Could you check a few things on this model? Use its own coordinates, in mm. Give positions to 0.01 mm unless a question says otherwise; leave off trailing zeros. Write each loop counter-clockwise with the first axis right and the second up, starting at its lowest first coordinate (ties: lowest second). Pieces come first, ordered by that corner, then holes. Notation, with made-up numbers: M -38.75,-17 L 16.25,-17 A13 cw 16.25,2 Z; hole C 51.25,77.25 d3. An arc over 180 degrees is marked long. Answer as a JSON object with one key per item and string values. Group by question number.
```python
from build123d import *

# Parameters (mm, degrees)
SKETCH1_W           = 60
SKETCH1_H           = 45
SKETCH1_R           = 2
BOSS_EXTRUDE1_DEPTH = 2
SKETCH2_R           = 12
CUT_EXTRUDE1_DEPTH  = 38.553295461


with BuildPart() as part:
    # Sketch1 → Boss-Extrude1 (new body)
    with BuildSketch(Plane(origin=(0, 0, 0), x_dir=(1, 0, 0), z_dir=(0, 1, 0))):
        Rectangle(SKETCH1_W, SKETCH1_H)
        with Locations(Location((-15.5, 15.5, 0), (0, 0, 270))):
            Circle(SKETCH1_R, mode=Mode.SUBTRACT)
        with Locations(Location((15.5, 15.5, 0), (0, 0, 270))):
            Circle(SKETCH1_R, mode=Mode.SUBTRACT)
        with Locations(Location((15.5, -15.5, 0), (0, 0, 270))):
            Circle(SKETCH1_R, mode=Mode.SUBTRACT)
        with Locations(Location((-15.5, -15.5, 0), (0, 0, 270))):
            Circle(SKETCH1_R, mode=Mode.SUBTRACT)
        with Locations(Location((-25.5, 15.5, 0), (0, 0, 270))):
            Circle(SKETCH1_R, mode=Mode.SUBTRACT)
        with Locations(Location((-25.5, -15.5, 0), (0, 0, 270))):
            Circle(SKETCH1_R, mode=Mode.SUBTRACT)
        with Locations(Location((25.5, -15.5, 0), (0, 0, 270))):
            Circle(SKETCH1_R, mode=Mode.SUBTRACT)
        with Locations(Location((25.5, 15.5, 0), (0, 0, 270))):
            Circle(SKETCH1_R, mode=Mode.SUBTRACT)
    extrude(amount=BOSS_EXTRUDE1_DEPTH)

    # Sketch2 → Cut-Extrude1 (cut, through all)
    with BuildSketch(Plane(origin=(0, 2, 0), x_dir=(1, 0, 0), z_dir=(0, 1, 0))):
        with Locations(Location((0, 0, 0), (0, 0, 270))):
            Circle(SKETCH2_R)
    extrude(amount=-CUT_EXTRUDE1_DEPTH, mode=Mode.SUBTRACT)


solid = part.part
```
1) If we section it at C-C, the plane z = 0: List the corners of the cut face in (x, y) for me.
2) Please list where these lines run through material, in increasing order: line 1 along X through (y, z) = (0.8, -15.5); line 2 along Z through (x, y) = (-25, 0.85); line 3 along Z through (x, y) = (-14.5, 0.8). Write a range as from..to.
3) If we section it at A-A, the plane x = 0: List the corners of the cut face in (y, z) for me.
4) If we section it at B-B, the plane z = 15.5: List the corners of the cut face in (x, y) for me, plus the area to 3 significant figures.
5) I'm going to push a flat-ended pin straight in: pin 1 (3 mm diameter, centred on x = 15.5, z = 15.5, fed in from +Y). Where does the tip first touch, or does it pass through?
6) If we section it at D-D, the plane x = 25.5: List the corners of the cut face in (y, z) for me.
7) We'd pull the mould along X, two halves only. Please class faces 1 (the flat face through (-7, 2, -10)), 2 (the cylindrical face through (-13.517, 0.986, -15.76)), 3 (the flat face through (30, 1, 0)), 4 (the cylindrical face through (-27.274, 0.986, 16.423)): released by +X, released by -X, zero draft, split by the parting line, or undercut.
Taken from the geometry:
{
 "1": {"outline": "M -30,0 L -12,0 L -12,2 L -30,2 Z; M 12,0 L 30,0 L 30,2 L 12,2 Z"},
 "2": {"line 1": "-30..-27.5, -23.5..-17.5, -13.5..13.5, 17.5..23.5, 27.5..30", "line 2": "-22.5..-17.44, -13.56..13.56, 17.44..22.5", "line 3": "-22.5..-17.23, -13.77..13.77, 17.23..22.5"},
 "3": {"outline": "M 0,-22.5 L 2,-22.5 L 2,-12 L 0,-12 Z; M 0,12 L 2,12 L 2,22.5 L 0,22.5 Z"},
 "4": {"outline": "M -30,0 L -27.5,0 L -27.5,2 L -30,2 Z; M -23.5,0 L -17.5,0 L -17.5,2 L -23.5,2 Z; M -13.5,0 L 13.5,0 L 13.5,2 L -13.5,2 Z; M 17.5,0 L 23.5,0 L 23.5,2 L 17.5,2 Z; M 27.5,0 L 30,0 L 30,2 L 27.5,2 Z", "area": "88.0 mm²"},
 "5": {"pin 1": "through"},
 "6": {"outline": "M 0,-22.5 L 2,-22.5 L 2,-17.5 L 0,-17.5 Z; M 0,-13.5 L 2,-13.5 L 2,13.5 L 0,13.5 Z; M 0,17.5 L 2,17.5 L 2,22.5 L 0,22.5 Z"},
 "7": {"face 1": "zero draft", "face 2": "undercut", "face 3": "released by +X", "face 4": "undercut"}
}
